The drawing under review shows one solid part. Ordinate dimensions are in mm from its lowest x, y, z. A direction names the side the tool comes from. Give positions to 0.01 mm unless a question says otherwise; leave off trailing zeros. Order: outer loops, then holes, each group sorted by start corner. A loop starts at its lowest first (then second) coordinate and runs counter-clockwise, first axis right, second up. Notation, with made-up numbers: M -40,34 L -7,34 A14 cw -7,53 Z; hole C 84.5,76.25 d8. An arc over 180 degrees is marked long. Put each result on its own line as item: value. Start each with the question number.
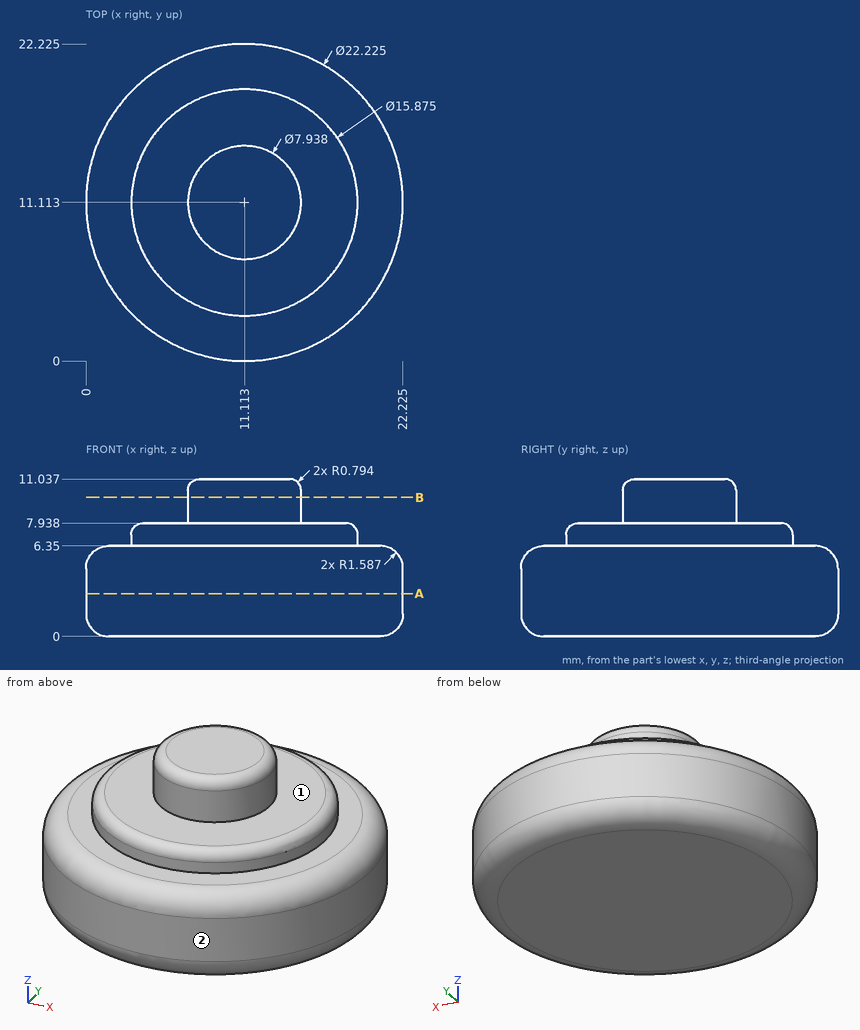
1. Consider section B-B on z = 9.75. Give the boundary of the cut face in (x, y).
2. To check wall thickness, follow probe 1 along Z at (x, y) = (19.5, 10.25); probe 2 along Z at (x, y) = (15.25, 14); probe 3 along Y at (x, z) = (13.5, 10.25) (1 decimal). State the ranges of each line that lie inside material, in increasing order.
3. Machinability: for the marked faces 1 and 2, which of the approach directions +Z, -Z, +X, -X, +Y, -Y give a long, thin tool a straight path to every point of the face, cutting with its end or side? Answer none if there is none.
4. Insertion check: pin 1 (5 mm diameter, centred on x = 4.5, z = 9, fed in from +Y); pin 2 (2 mm diameter, centred on y = 9.5, z = 2, fed in from -X); pin 3 (8 mm diameter, centred on x = 5.5, y = 19, fed in from +Z). Each pin has a flat end and moves straight along its axis. Give the tip position at first contact, or say it passes through.
5. Consider section A-A on z = 3. Give the boundary of the cut face in (x, y) (1 decimal), then the cut area to 3 significant figures.
Returned:
1. outline: C 11.11,11.11 d7.94
2. probe 1: z = 0 to 6.35
2. probe 2: z = 0 to 7.94
2. probe 3: y = 7.9 to 14.3
3. face 1: +Z
3. face 2: +Z, -Z
4. pin 1: stops at y = 17.47
4. pin 2: stops at x = 0.02
4. pin 3: stops at z = 7.94
5. outline: C 11.1,11.1 d22.2
5. area: 388 mm2
